Autodesk Inventor part; units mm, degrees
ref_plane "YZ Plane" through (0, 0, 0) normal (1, 0, 0) x (0, 1, 0)
ref_plane "XZ Plane" through (0, 0, 0) normal (0, 1, 0) x (-1, 0, 0)
ref_plane "XY Plane" through (0, 0, 0) normal (0, 0, 1) x (1, 0, 0)
sketch "スケッチ1" plane through (0, 0, 0) normal (0, 0, 1) x (1, 0, 0)
  line L0 (-27.5, 43.5) -> (27.5, 43.5)
  line L1 (27.5, 43.5) -> (27.5, -43.5)
  line L2 (27.5, -43.5) -> (-27.5, -43.5)
  line L3 (-27.5, -43.5) -> (-27.5, 43.5)
  point P0 (0, 0)
  dimension "d0" = 87
  dimension "d1" = 55
  dimension "d2" = 27.5
  dimension "d3" = 43.5
extrude "押し出し1" add sketch "スケッチ1" along normal blind 3
sketch "スケッチ2" plane through (0, 0, 3) normal (0, 0, 1) x (1, 0, 0)
  circle A0 centre (-24.25, 28.5) radius 1.6
  circle A1 centre (24.25, 28.5) radius 1.6
  circle A2 centre (-21, -37.5) radius 1.6
  circle A3 centre (21, -37.5) radius 1.6
  line L0 (-27.5, 43.5) -> (27.5, 43.5)
  point P0 (0, 0)
  dimension "d6" = 3.2
  dimension "d7" = 48.5
  dimension "d8" = 42
  dimension "d9" = 21
  dimension "d10" = 24.25
  dimension "d11" = 66
  dimension "d12" = 66
  dimension "d22" = 15
  dimension "d23" = 15
hole "穴1" at (-21, -37.5, 3) at (21, -37.5, 3) at (24.25, 28.5, 3) at (-24.25, 28.5, 3) direction (0, 0, -1) diameter 3.2 end through all
sketch "スケッチ3" plane through (0, 0, 3) normal (0, 0, 1) x (1, 0, 0)
  line L0 (27.5, -43.5) -> (-27.5, -43.5)
  line L1 (-26.5, 24.5) -> (-21.5, 24.5)
  line L2 (-21.5, 24.5) -> (-21.5, -34.5)
  line L3 (-21.5, -34.5) -> (-26.5, -34.5)
  line L4 (-26.5, -34.5) -> (-26.5, 24.5)
  line L5 (21.5, 24.5) -> (26.5, 24.5)
  line L6 (26.5, 24.5) -> (26.5, -34.5)
  line L7 (26.5, -34.5) -> (21.5, -34.5)
  line L8 (21.5, -34.5) -> (21.5, 24.5)
  point P0 (0, 0)
  dimension "d24" = 5
  dimension "d25" = 59
  dimension "d26" = 9
  dimension "d27" = 9
  dimension "d28" = 43
  dimension "d29" = 21.5
extrude "押し出し2" add sketch "スケッチ3" along normal blind 8.5
sketch "スケッチ4" plane through (0, 0, 3) normal (0, 0, 1) x (1, 0, 0)
  line L0 (-5.5, 25) -> (10.5, 25)
  line L1 (10.5, 25) -> (10.5, 46)
  line L2 (10.5, 46) -> (-5.5, 46)
  line L3 (-5.5, 46) -> (-5.5, 25)
  line L4 (27.5, 43.5) -> (27.5, -43.5)
  point P0 (0, 0)
  dimension "d57" = 16
  dimension "d58" = 21
  dimension "d59" = 2.5
  dimension "d60" = 17
extrude "押し出し3" add sketch "スケッチ4" along normal blind 13.5
sketch "スケッチ5" plane through (0, 0, 3) normal (0, 0, 1) x (1, 0, 0)
  line L0 (-22.5, 46) -> (-13.5, 46)
  line L1 (-13.5, 46) -> (-13.5, 32)
  line L2 (-13.5, 32) -> (-22.5, 32)
  line L3 (-22.5, 32) -> (-22.5, 46)
  line L4 (-27.5, -43.5) -> (-27.5, 43.5)
  point P0 (5.6589, 43.5)
  dimension "d61" = 5
  dimension "d62" = 9
  dimension "d63" = 14
  dimension "d64" = 2.5
extrude "押し出し4" add sketch "スケッチ5" along normal blind 11
sketch "スケッチ6" plane through (0, 0, 3) normal (0, 0, 1) x (1, 0, 0)
  line L0 (27.5, -43.5) -> (-27.5, -43.5)
  line L1 (-17.5, -43.5) -> (-4.5, -43.5)
  line L2 (-4.5, -43.5) -> (-4.5, -29)
  line L3 (-4.5, -29) -> (-17.5, -29)
  line L4 (-17.5, -29) -> (-17.5, -43.5)
  line L5 (-27.5, -43.5) -> (-27.5, 43.5)
  point P0 (0, 0)
  dimension "d65" = 13
  dimension "d66" = 10
  dimension "d67" = 14.5
extrude "押し出し5" add sketch "スケッチ6" along normal blind 7
sketch "スケッチ7" plane through (0, 0, 0) normal (0, 0, -1) x (-1, 0, 0)
  line L0 (5.5, -44.5) -> (-0.5, -44.5)
  line L1 (-0.5, -44.5) -> (-0.5, -36.5)
  line L2 (-0.5, -36.5) -> (5.5, -36.5)
  line L3 (5.5, -36.5) -> (5.5, -44.5)
  line L4 (27.5, -43.5) -> (27.5, 43.5)
  point P0 (0, 0)
  dimension "d68" = 6
  dimension "d69" = 8
  dimension "d70" = 22
  dimension "d71" = 1
extrude "押し出し6" add sketch "スケッチ7" along normal blind 3
sketch "スケッチ8" plane through (0, 0, 0) normal (0, 0, -1) x (-1, 0, 0)
  line L0 (-27.5, -43.5) -> (-0.5, -43.5)
  line L1 (-3.5, -43.5) -> (-17.5, -43.5)
  line L2 (-17.5, -43.5) -> (-17.5, -28.5)
  line L3 (-17.5, -28.5) -> (-3.5, -28.5)
  line L4 (-3.5, -28.5) -> (-3.5, -43.5)
  line L5 (-27.5, 43.5) -> (-27.5, -43.5)
  point P0 (0, 0)
  dimension "d72" = 14
  dimension "d73" = 15
  dimension "d74" = 10
extrude "押し出し7" add sketch "スケッチ8" along normal blind 1.5
sketch "スケッチ9" plane through (0, 0, 0) normal (0, 0, -1) x (-1, 0, 0)
  line L0 (-21, 44.5) -> (-13, 44.5)
  line L1 (-13, 44.5) -> (-13, 37.5)
  line L2 (-13, 37.5) -> (-21, 37.5)
  line L3 (-21, 37.5) -> (-21, 44.5)
  line L4 (-27.5, 43.5) -> (-27.5, -43.5)
  point P0 (0, 0)
  dimension "d75" = 8
  dimension "d76" = 7
  dimension "d77" = 6.5
  dimension "d78" = 1
extrude "押し出し8" add sketch "スケッチ9" along normal blind 4
sketch "スケッチ11" plane through (0, 0, 3) normal (0, 0, 1) x (1, 0, 0)
  line L0 (-20.5, 1.5) -> (-18, 1.5)
  line L1 (-18, 1.5) -> (-18, -13.5)
  line L2 (-18, -13.5) -> (-20.5, -13.5)
  line L3 (-20.5, -13.5) -> (-20.5, 1.5)
  line L4 (-17.5, -43.5) -> (-27.5, -43.5)
  line L5 (-21.5, 24.5) -> (-21.5, -34.5)
  point P0 (0, 0)
  dimension "d79" = 15
  dimension "d80" = 2.5
  dimension "d81" = 30
  dimension "d82" = 1
extrude "押し出し10" add sketch "スケッチ11" along normal blind 8.5
sketch "スケッチ12" plane through (0, 0, 3) normal (0, 0, 1) x (1, 0, 0)
  line L0 (-19.5, -17) -> (-13.5, -17)
  line L1 (-13.5, -17) -> (-13.5, -23.5)
  line L2 (-13.5, -23.5) -> (-19.5, -23.5)
  line L3 (-19.5, -23.5) -> (-19.5, -17)
  line L4 (-17.5, -43.5) -> (-27.5, -43.5)
  line L5 (-21.5, 24.5) -> (-21.5, -34.5)
  point P0 (0, 0)
  dimension "d83" = 6
  dimension "d84" = 6.5
  dimension "d86" = 2
  dimension "d87" = 20
extrude "押し出し11" add sketch "スケッチ12" along normal blind 5
sketch "スケッチ13" plane through (0, 0, 14) normal (0, 0, 1) x (1, 0, 0)
  line L0 (-13.5, 46) -> (-13.5, 32)
  line L1 (-22.5, 32) -> (-13.5, 32)
  line L2 (-13.5, 32) -> (-13.5, 43)
  line L3 (-13.5, 43) -> (-22.5, 43)
  line L4 (-22.5, 43) -> (-22.5, 32)
  point P0 (0, 0)
  dimension "d112" = 11
extrude "押し出し13" cut sketch "スケッチ13" against normal blind 1
sketch "スケッチ14" plane through (0, 0, 3) normal (0, 0, 1) x (1, 0, 0)
  line L0 (-17.5, -43.5) -> (-27.5, -43.5)
  line L1 (-21.5, 24.5) -> (-21.5, -34.5)
  line L2 (-19.5, -25.5) -> (-12.5, -25.5)
  line L3 (-12.5, -25.5) -> (-12.5, -27.5)
  line L4 (-12.5, -27.5) -> (-19.5, -27.5)
  line L5 (-19.5, -27.5) -> (-19.5, -25.5)
  point P0 (0, 0)
  dimension "d88" = 7
  dimension "d89" = 2
  dimension "d90" = 2
  dimension "d91" = 16
extrude "押し出し14" add sketch "スケッチ14" along normal blind 9
sketch "スケッチ10" plane through (0, 0, 3) normal (0, 0, 1) x (1, 0, 0)
  line L0 (-5.5, 5.5) -> (9.5, 5.5)
  line L1 (9.5, 5.5) -> (9.5, -9.5)
  line L2 (9.5, -9.5) -> (-5.5, -9.5)
  line L3 (-5.5, -9.5) -> (-5.5, 5.5)
  line L4 (-9.5, -16.5) -> (4.5, -16.5)
  line L5 (4.5, -16.5) -> (4.5, -25.5)
  line L6 (4.5, -25.5) -> (-9.5, -25.5)
  line L7 (-9.5, -25.5) -> (-9.5, -16.5)
  line L8 (9.5, 20.5) -> (20.5, 20.5)
  line L9 (20.5, 20.5) -> (20.5, 7.5)
  line L10 (20.5, 7.5) -> (9.5, 7.5)
  line L11 (9.5, 7.5) -> (9.5, 20.5)
  line L12 (27.5, -43.5) -> (-4.5, -43.5)
  line L13 (27.5, 43.5) -> (27.5, -43.5)
  line L14 (10.5, 43.5) -> (27.5, 43.5)
  line L15 (8.5, -16.5) -> (17.5, -16.5)
  line L16 (17.5, -16.5) -> (17.5, -25.5)
  line L17 (17.5, -25.5) -> (8.5, -25.5)
  line L18 (8.5, -25.5) -> (8.5, -16.5)
  point P0 (0, 0)
  dimension "d94" = 11
  dimension "d95" = 15
  dimension "d96" = 14
  dimension "d97" = 9
  dimension "d98" = 9
  dimension "d99" = 9
  dimension "d100" = 15
  dimension "d101" = 13
  dimension "d102" = 23
  dimension "d103" = 38
  dimension "d104" = 18
  dimension "d105" = 18
  dimension "d106" = 7
  dimension "d107" = 18
  dimension "d108" = 10
  dimension "d109" = 4
extrude "押し出し15" add sketch "スケッチ10" along normal blind 1
fillet "フィレット1" radius 4 2 edges at (-13.5, 37.5, 13) (-22.5, 37.5, 13)
properties part number "43" material "PC/ABS プラスチック"
Part model, mm, in its own coordinate system. A direction names the side the tool comes from. Coordinates: 2 decimals unless noted, no trailing zeros. Loops run counter-clockwise (first coordinate to the right, second up) from the corner with the lowest first, then second, coordinate; pieces in that order, holes last. Notation, with made-up numbers: M 78.25,32.25 L 107.25,32.25 A21 ccw 107.25,49.25 Z; hole C -28,79.5 d6. An arc over 180 degrees is marked long. Use a Markdown table: item, result. Add a question column.
Q1. Which spindle directions (+Z, -Z, +X, -X, +Y, -Y) get a long thin tool onto all of the face, cutting with end or side? Do faces 1 (the flat face through (21.5, -5, 7)), 2 (the flat face through (-16, -23.5, 5)), 3 (the flat face through (-19, -6, 11.5)). Say none if no direction does.
Q2. Pin check, flat tips, straight feed: P1, Ø4, axis at y = -15, z = 6.5, coming from the +X side; P2, Ø5.5, axis at x = -15.5, z = 6.5, coming from the -Y side; P3, Ø5, axis at x = 19, y = -35, coming from the +Z side. Stop position of each tip, or through.
Q3. Mould opens along Y. For faces 4 (the flat face through (-2, -36.5, -1)), 5 (the flat face through (2, 36, 16.5)), 6 (the cylindrical face through (-22.586, -37.292, 1.479)) say: +Y half, -Y half, draft (parallel to the pull), parting line (faces both ways), or undercut.
Q4. Probe L1, parallel to X at y = -37.5, z = 1.85; L2, parallel to X at y = 28.5, z = 0.7; L3, parallel to Y at x = -24.25, z = 1.45. List the from-to ranges inside material, lowest first.
Q5. Cut at B-B (x = 24.25). Write the cut outline in (y, z).
Q6. Cut at A-A (z = 6.5). Give the number of separate pieces and of enclosed holes in the cut face, and give its area (3 significant figures).
Q7. Cut at C-C (y = -37.5). Write the cut outline in (x, z), and give its area (3 significant figures).
Q8. Cut at D-D (x = -3). Write the cut outline in (y, z), and give its area (4 significant figures).
Worked out:
| question | item | result |
|---|---|---|
| 1 | face 1 | +Z, +Y, -Y |
| 1 | face 2 | +Z |
| 1 | face 3 | +Z, +X, -X |
| 2 | P1 | stops at x = 26.5 |
| 2 | P2 | stops at y = -43.5 |
| 2 | P3 | stops at z = 3 |
| 3 | face 4 | +Y half |
| 3 | face 5 | draft |
| 3 | face 6 | undercut |
| 4 | L1 | x = -27.5 to -22.6, -19.4 to 19.4, 22.6 to 27.5 |
| 4 | L2 | x = -27.5 to -25.85, -22.65 to 22.65, 25.85 to 27.5 |
| 4 | L3 | y = -43.5 to 26.9, 30.1 to 43.5 |
| 5 | outline | M -43.5,0 L 26.9,0 L 26.9,3 L 24.5,3 L 24.5,11.5 L -34.5,11.5 L -34.5,3 L -43.5,3 Z; M 30.1,0 L 43.5,0 L 43.5,3 L 30.1,3 Z |
| 6 | separate pieces | 8 |
| 6 | enclosed holes | 0 |
| 6 | area | 1,330 mm2 |
| 7 | outline | M -27.5,0 L -22.6,0 L -22.6,3 L -27.5,3 Z; M -19.4,0 L -5.5,0 L -5.5,-3 L 0.5,-3 L 0.5,0 L 3.5,0 L 3.5,-1.5 L 17.5,-1.5 L 17.5,0 L 19.4,0 L 19.4,3 L -4.5,3 L -4.5,10 L -17.5,10 L -17.5,3 L -19.4,3 Z; M 22.6,0 L 27.5,0 L 27.5,3 L 22.6,3 Z |
| 7 | area | 276 mm2 |
| 8 | outline | M -44.5,-3 L -36.5,-3 L -36.5,0 L 43.5,0 L 43.5,3 L 46,3 L 46,16.5 L 25,16.5 L 25,3 L 5.5,3 L 5.5,4 L -9.5,4 L -9.5,3 L -16.5,3 L -16.5,4 L -25.5,4 L -25.5,3 L -43.5,3 L -43.5,0 L -44.5,0 Z |
| 8 | area | 592.5 mm2 |
